```python
from build123d import *

# Parameters (mm, degrees)
BOSS_EXTRUDE1_DEPTH = 10
TAPPED_HOLE1_D      = 4.134


with BuildPart() as part:
    # Sketch1 → Boss-Extrude1 (new body)
    with BuildSketch(Plane(origin=(-5, 0, 0), x_dir=(0, 0, -1), z_dir=(1, 0, 0))):
        Polygon((4, -1.7), (-4, -1.7), (-5, -2.7), (-5, -3.7), (5, -3.7), (5, -2.7), align=None)
    extrude(amount=BOSS_EXTRUDE1_DEPTH)

    # Sketch2 → Revolve1 (revolve)
    with BuildSketch(Plane(origin=(0, 0, 0), x_dir=(0, 0, -1), z_dir=(1, 0, 0))):
        Polygon((3.35, -1.7), (3, 0), (0, 0), (0, -1.7), align=None)
    revolve(axis=Axis((0, 0, 0), (0, -1, 0)))

    # Tapped Hole1 (through all)
    with Locations(Plane(origin=(0, 0, 0), x_dir=(1, 0, 0), z_dir=(0, 1, 0))):
        with Locations((0, 0)):
            Hole(TAPPED_HOLE1_D / 2)


solid = part.part
```
Input: part model. Units: mm. Frame: model coordinates. A direction names the side the tool comes from. Round coordinates to 2 decimals unless told otherwise and drop trailing zeros. Write each loop counter-clockwise with the first axis right and the second up, starting at its lowest first coordinate (ties: lowest second). Pieces come first, ordered by that corner, then holes. Notation, with made-up numbers: (68, -0.75) - (103, -0.75) arc R21 cw to (103, 23.25) - close; hole circle Ø7 at (47, 40.5). An arc over 180 degrees is marked (long way). Write item = value, one per line.
(1) Access query for faces 1 (the flat face through (0, -3, 5)), 2 (the flat face through (-3.4, -1.7, -0.9)). Directions: +Z, -Z, +X, -X, +Y, -Y. A direction counts if a zero-diameter tool reaches every point of the face in a straight line with its end or side. Return the directions, or none.
Geometry check:
face_1 = +Z, +X, -X, +Y, -Y
face_2 = +Y
(2) Material intervals for probe 1 along Z at (x, y) = (0, -1.8); probe 2 along Y at (x, z) = (4, -0.25); probe 3 along Z at (x, y) = (0, -1.15), sorted ascending.
Geometry check:
probe_1 = -4.1 to -2.07, 2.07 to 4.1
probe_2 = -3.7 to -1.7
probe_3 = -3.24 to -2.07, 2.07 to 3.24
(3) Section query B-B on z = 0. Output: boundary loops of the cut face in (x, y).
Geometry check:
outline = (-5, -3.7) - (-2.07, -3.7) - (-2.07, 0) - (-3, 0) - (-3.35, -1.7) - (-5, -1.7) - close; (2.07, -3.7) - (5, -3.7) - (5, -1.7) - (3.35, -1.7) - (3, 0) - (2.07, 0) - close
(4) Contact query for a flat-ended pin moving along its axis: pin 1 Ø1.5 at (x, y) = (-1, -2) entering from -Z. Output: stop coordinate, or through.
Geometry check:
pin_1 = -5
(5) Section query A-A on x = 0. Output: boundary loops of the cut face in (y, z).
Geometry check:
outline = (-3.7, -5) - (-2.7, -5) - (-1.7, -4) - (-1.7, -3.35) - (0, -3) - (0, -2.07) - (-3.7, -2.07) - close; (-3.7, 2.07) - (0, 2.07) - (0, 3) - (-1.7, 3.35) - (-1.7, 4) - (-2.7, 5) - (-3.7, 5) - close
(6) Pull-direction query (X, two-part tool) for faces 3 (the flat face through (-0.1, -2.2, -4.5)), 4 (the cylindrical face through (1.64, -1.88, 1.26)), 5 (the conical face through (-1.9, -0.3, 2.4)); classes: +X half, -X half, draft (parallel to the pull), parting line (faces both ways), or undercut.
Geometry check:
face_3 = draft
face_4 = undercut
face_5 = parting line
(7) Section query C-C on y = -2.9. Output: boundary loops of the cut face in (x, z), then the cut area to 3 significant figures.
Geometry check:
outline = (-5, -5) - (5, -5) - (5, 5) - (-5, 5) - close; hole circle Ø4.13 at (0, 0)
area = 86.6 mm^2
(8) Section query D-D on x = 4.25. Output: boundary loops of the cut face in (y, z), then the cut area to 3 significant figures.
Geometry check:
outline = (-3.7, -5) - (-2.7, -5) - (-1.7, -4) - (-1.7, 4) - (-2.7, 5) - (-3.7, 5) - close
area = 19.0 mm^2
